Could you check a few things on this model? Use its own coordinates, in mm. A direction names the side the tool comes from. Round coordinates to 2 decimals unless told otherwise and drop trailing zeros. Write each loop counter-clockwise with the first axis right and the second up, starting at its lowest first coordinate (ties: lowest second). Pieces come first, ordered by that corner, then holes. Notation, with made-up numbers: M 55.5,25.25 L 84.5,25.25 A22 cw 84.5,43.25 Z; hole C 10,41 d9. An arc over 180 degrees is marked long. One line per item, written item: value. Start each with the question number.
(1) I want a section at C-C on z = 20. Please give me the cut outline in (x, y).
(2) I want a section at B-B on x = 72.5. Please give me the cut outline in (y, z), and give its area (3 significant figures).
(3) If I drill on L1, parallel to Z at x = 33, y = -7.5; L2, parallel to Z at x = 61.5, y = -3.5; L3, parallel to X at y = -42.5, z = 12.5, over which ranges is the centre line in solid material (lowest first)?
(4) I want a section at A-A on y = -65. Please give me the cut outline in (x, z), and give its area (3 significant figures).
(5) Which directions (+Z, -Z, +X, -X, +Y, -Y) give clear straight access to the entire face, cutting with the end or side of a thin tool? Please do faces 1 (the face through (44.799, -49, 43)), 2 (the face through (30, -49, 45)), 3 (the face through (29.799, -49, 17)).
(6) I'm going to push flat-ended pins straight in: pin 1 Ø1.2 at (y, z) = (-74, 26.5) entering from +X; pin 2 Ø10 at (x, y) = (59, -65.5) entering from +Z. Where does each tip first touch, or does it pass through?
(7) Thinking about a two-plate mould opening in Z: for faces 4 (the face through (7.503, -49.3, 35.14)), 5 (the face through (88, -49, 5)), 6 (the face through (59, -49, 10)), 7 (the face through (37, -49, 25)), which applies, released by +Z, released by -Z, zero draft, split by the parting line, or undercut?
```python
from build123d import *

# Parameters (mm, degrees)
F1_DEPTH = 100


with BuildPart() as f1:
    # F0 (on Front) → F1 (new body)
    with BuildSketch(Plane.XZ):
        with BuildLine():
            Line((0, 25), (0, 0))
            Line((0, 0), (88, 0))
            Line((88, 0), (88, 10))
            Line((88, 10), (29.799222, 10))
            Line((29.799222, 10), (29.799222, 25))
            Line((29.799222, 25), (44.799222, 25))
            Line((44.799222, 25), (44.799222, 29))
            ThreePointArc((44.799222, 29), (38.799222, 35), (44.799222, 41))
            Line((44.799222, 41), (44.799222, 45))
            Line((44.799222, 45), (14.799222, 45))
            Line((14.799222, 45), (0, 25))
        make_face()
        with BuildLine():
            ThreePointArc((50.799222, 35), (49.041862, 39.242641), (44.799222, 41))
            ThreePointArc((44.799222, 41), (38.799222, 35), (44.799222, 29))
            ThreePointArc((44.799222, 29), (49.041862, 30.757359), (50.799222, 35))
        make_face()
    extrude(amount=F1_DEPTH)


solid = f1.part
```
Found:
1. outline: M 0,-100 L 29.8,-100 L 29.8,0 L 0,0 Z
2. outline: M -100,0 L 0,0 L 0,10 L -100,10 Z
2. area: 1,000 mm²
3. L1: z = 0 to 10, 25 to 45
3. L2: z = 0 to 10
3. L3: x = 0 to 29.8
4. outline: M 0,0 L 88,0 L 88,10 L 29.8,10 L 29.8,25 L 44.8,25 L 44.8,29 A6 ccw 50.8,35 A6 ccw 44.8,41 L 44.8,45 L 14.8,45 L 0,25 Z
4. area: 2,130 mm²
5. face 1: +Z, +X, +Y, -Y
5. face 2: +Z, +X, -X, +Y, -Y
5. face 3: +X, +Y, -Y
6. pin 1: stops at x = 44.8
6. pin 2: stops at z = 10
7. face 4: released by +Z
7. face 5: zero draft
7. face 6: undercut
7. face 7: undercut
